Model file for the job. Use its own axes, mm. A direction names the side the tool comes from. Round coordinates to 2 decimals unless told otherwise and drop trailing zeros. Loops run counter-clockwise (first coordinate to the right, second up) from the corner with the lowest first, then second, coordinate; pieces in that order, holes last. Notation, with made-up numbers: M 12,-17.5 L 66,-17.5 A19 ccw 66,-7.5 Z; hole C -24.75,-12 d7. An arc over 180 degrees is marked long. Use a Markdown table: item, result. Add a question column.
Q1. Cut at A-A (x = 6). Give the cut face in (y, z), plus the area to 3 significant figures.
Q2. Cut at C-C (z = 89). Give the cut face in (x, y), plus the area to 3 significant figures.
Q3. Cut at D-D (x = -18). Give the cut face in (y, z), plus the area to 3 significant figures.
Q4. Mould opens along Y. For faces 4 (the face through (30, -97, 1)), 5 (the face through (-10.37, 3.86, -127.16)), 6 (the face through (-27, 100, -39)) say: +Y half, -Y half, draft (parallel to the pull), parting line (faces both ways), or undercut.
Q5. Probe line 1 (X direction, y = -7.5, z = 87); line 2 (Y direction, x = -14.5, z = 143); line 3 (Y direction, x = -13.5, z = -110.5). List the from-to ranges inside material, lowest first. Write a range as from..to.
Q6. Pin check, flat tips, straight feed: pin 1 (12 mm diameter, centred on x = 15.5, z = 40.5, fed in from +Y); pin 2 (1 mm diameter, centred on x = -19.5, y = -25, fed in from +Z); pin 3 (10 mm diameter, centred on y = 0, z = -127.5, fed in from +X). Stop position of each tip, or through.
Q7. Tool access for faces 1 (the face through (2.12, 21.47, -22.33)), 2 (the face through (2.115, 14.273, -25.559)), 3 (the face through (2, -95, 7)): list every direction of +Z, -Z, +X, -X, +Y, -Y with a clear straight run to the whole face (end or side of a thin tool).
Q8. Cut at B-B (y = -55). Give the cut face in (x, z).
Autodesk Inventor part; units mm, degrees
ref_plane "YZ Plane" through (0, 0, 0) normal (1, 0, 0) x (0, 1, 0)
ref_plane "XZ Plane" through (0, 0, 0) normal (0, 1, 0) x (-1, 0, 0)
ref_plane "XY Plane" through (0, 0, 0) normal (0, 0, 1) x (1, 0, 0)
sketch "スケッチ1" plane through (0, 0, 0) normal (1, 0, 0) x (0, 1, 0)
  line L0 (100, 200) -> (-100, 200)
  line L1 (-100, 200) -> (-100, -200)
  line L2 (-100, -200) -> (100, -200)
  line L3 (100, -200) -> (100, 200)
  line L4 (-140, 0) -> (140, 0)
  line L5 (0, -280) -> (0, 280)
  point P0 (0, 0)
  point P1 (100, 0)
  point P2 (0, 200)
  dimension "d2" = 200
  dimension "d3" = 400
extrude "押し出し1" add sketch "スケッチ1" along normal mid plane 60
sketch "スケッチ3" plane through (-30, 100, 200) normal (0, 1, 0) x (1, 0, 0)
  line L0 (0, 0) -> (60, 0)
  line L1 (60, 0) -> (5, 0)
  line L2 (60, 392) -> (60, 0)
  line L3 (60, 400) -> (60, 0)
  line L4 (5, 0) -> (5, 250)
  arc A0 (60, 392) -> (5, 250) centre (215.8091, 250) ccw
  line L5 (0, 0) -> (0, 400)
  line L6 (0, 400) -> (60, 400)
  arc A1 (60, 400) -> (0, 264.2446) centre (215.8091, 250) ccw
  dimension "d16" = 5
  dimension "d18" = 250
  dimension "d21" = 8
extrude "押し出し2" cut sketch "スケッチ3" against normal through all contours L4 A0 L2 L0 | L5 L6 A1
sketch "スケッチ7" plane through (-25, 100, 200) normal (1, 0, 0) x (0, 0, -1)
  arc A0 (50, -130) -> (350, 0) centre (-43.1737, 496.1701) ccw
  arc A1 (50, -130) -> (350, 0) centre (25.3027, 338.1476) ccw
  line L0 (50, -130) -> (350, 0)
  line L1 (0, -200) -> (0, 0)
  line L2 (0, 0) -> (250, 0)
  line L3 (400, -200) -> (400, 0)
  dimension "d30" = 50
  dimension "d31" = 130
  dimension "d38" = 50
extrude "押し出し5" add sketch "スケッチ7" along normal blind 55 contours A0 A1
sketch "スケッチ8" plane through (0, 0, 0) normal (0, 1, 0) x (-1, 0, 0)
  line L0 (-30, -200) -> (-30, -192)
  line L1 (-30, -200) -> (30, -200)
  line L2 (30, 200) -> (30, -64.2446)
  arc A0 (-30, -200) -> (30, -64.2446) centre (-185.8091, -50) ccw
  arc A1 (-30, -200) -> (-30, -200) centre (-53.5814, -108.4409) ccw
  line L3 (30, -200) -> (30, -64.2446)
  point P0 (0, 0)
extrude "押し出し6" cut sketch "スケッチ8" along normal through all contours A1 L3 L1 | A0 L3 A1
fillet "フィレット2" radius 1 1 edges at (15.1138, 100, -150)
fillet "フィレット2" radius 2 1 edges at (2.5, -30, 150)
sketch "スケッチ10" plane through (-30, -100, -64.2446) normal (0, -1, 0) x (1, 0, 0)
  line L0 (0, 264.2446) -> (5, 264.2446)
  line L1 (5, 264.2446) -> (60, 264.2446)
  arc A0 (5, 14.2446) -> (60, -127.7554) centre (215.8091, 14.2446) ccw
  line L2 (60, 264.2446) -> (60, -127.7554)
  line L3 (5, 14.2446) -> (5, 264.2446)
  line L4 (5, 264.2446) -> (5, 14.2446)
  line L5 (0, 264.2446) -> (0, 0)
  point P0 (30, 64.2446)
extrude "押し出し7" add sketch "スケッチ10" against normal blind 5
fillet "フィレット3" radius 50 1 edges at (-27.5, 100, 200)
properties part number "type8_end_plate" material "CFRP"
Checked values:
| question | item | result |
|---|---|---|
| 1 | outline | M -100,-170.19 L 100,-170.19 L 100,-160.04 L -95,-160.04 L -95,200 L -100,200 Z; M -24.82,100.99 A468.8 ccw 84.78,-133.37 A1 ccw 86.34,-132.12 A633.06 cw -20.9,101.75 A2 ccw Z |
| 1 | area | 5,470 mm^2 |
| 2 | outline | M -30,-100 L 30,-100 L 30,-95 L -25,-95 L -25,-22.75 L 30,-22.75 L 30,-17.83 L -25,-17.83 L -25,100 L -30,100 Z |
| 2 | area | 1,550 mm^2 |
| 3 | outline | M -100,-122.38 L 100,-122.38 L 100,-103.87 L 66.71,-103.87 A633.06 cw -20.9,101.75 A2 ccw -24.82,100.99 A468.8 ccw 61.09,-103.87 L -95,-103.87 L -95,200 L -100,200 Z |
| 3 | area | 6,740 mm^2 |
| 4 | face 4 | draft |
| 4 | face 5 | undercut |
| 4 | face 6 | +Y half |
| 5 | line 1 | x = -30..-25 |
| 5 | line 2 | y = -100..-95 |
| 5 | line 3 | y = -100..-95, 66.08..71.11 |
| 6 | pin 1 | stops at y = -1.51 |
| 6 | pin 2 | stops at z = 102.43 |
| 6 | pin 3 | stops at x = -8.19 |
| 7 | face 1 | +Z, +X, +Y |
| 7 | face 2 | +X |
| 7 | face 3 | +Z, +X |
| 8 | outline | M -30,-64.24 A216.28 ccw 30,-200 L 30,-192 A210.81 cw -25,-50 L -25,200 L -30,200 Z |
